Verification items for the finished model (mm, model axes). Face numbers are marked on the shaded views. A direction names the side the tool comes from. Give positions to 0.01 mm unless a question says otherwise; leave off trailing zeros.
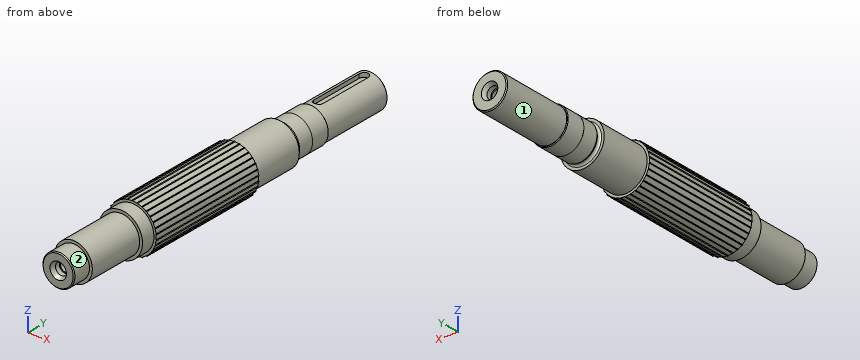
from build123d import *

# Parameters (mm, degrees)
F3_DEPTH        = 235.8934182005
F3_COPIES_COUNT = 30
F6_DEPTH        = 5
F7_SIZE         = 1.016
F10_D           = 10.5
F10_DEPTH       = 31.9574
F10_TIP         = 3.1545182499
F11_SIZE        = 0.762
F14_D           = 10.5
F14_DEPTH       = 31.9532
F14_TIP         = 3.1545182499


# Not quite as in the source:
# - a pattern or mirror of a feature is missing from the dataset's text; its kind, count and spacing are read off the source's solid


with BuildPart() as f1:
    # F0 (on Right) → F1 (revolve)
    with BuildSketch(Plane.YZ):
        with BuildLine():
            Line((59.3317817995, 23.876), (2.032, 23.876))
            Line((2.032, 23.876), (2.032, 27.1526))
            Line((2.032, 27.1526), (0, 27.1526))
            Line((0, 27.1526), (-135, 27.1526))
            Line((-135, 27.1526), (-135, 23.876))
            Line((-135, 23.876), (-150.24, 23.876))
            Line((-150.24, 23.876), (-150.24, 20.6375))
            Line((-150.24, 20.6375), (-213.3880182005, 20.6375))
            Line((-213.3880182005, 20.6375), (-213.3880182005, 17.5006))
            Line((-213.3880182005, 17.5006), (-233.8604182005, 17.5006))
            Line((-233.8604182005, 17.5006), (-233.8604182005, 9.0551))
            Line((-233.8604182005, 9.0551), (-229.4662182005, 6.5024))
            Line((-229.4662182005, 6.5024), (-224.3608182005, 6.5024))
            Line((-224.3608182005, 6.5024), (-224.3608182005, 0))
            Line((-224.3608182005, 0), (174.0127817995, 0))
            Line((174.0127817995, 0), (174.0127817995, 6.5024))
            Line((174.0127817995, 6.5024), (179.1181817995, 6.5024))
            Line((179.1181817995, 6.5024), (183.5123817995, 9.0551))
            Line((183.5123817995, 9.0551), (183.5123817995, 18.9992))
            Line((183.5123817995, 18.9992), (103.5023817995, 18.9992))
            Line((103.5023817995, 18.9992), (103.5023817995, 19.97075))
            Line((103.5023817995, 19.97075), (81.7853817995, 19.97075))
            Line((81.7853817995, 19.97075), (81.7853817995, 20.00758))
            Line((81.7853817995, 20.00758), (64.3216122695, 20.00758))
            Line((64.3216122695, 20.00758), (62.6845817995, 19.0624400175))
            ThreePointArc((62.6845817995, 19.0624400175), (60.4493817995, 19.0624400175), (59.3317817995, 20.99818))
            Line((59.3317817995, 20.99818), (59.3317817995, 23.876))
        make_face()
    revolve(axis=Axis((0, -25.1740182005, 0), (0, 1, 0)))

    # F2 (on face) → F3 (cut, through all)
    with BuildSketch(Plane(origin=(0, 2.032, 0), x_dir=(-1, 0, 0), z_dir=(0, 1, 0))):
        with BuildLine():
            Line((-0.442078818, 26.3868970263), (0, 27.1526))
            ThreePointArc((0, 27.1526), (-2.8382195517, 27.0038552162), (-5.6453429761, 26.5592505437))
            Line((-5.6453429761, 26.5592505437), (-5.0537260411, 25.9021933716))
            ThreePointArc((-5.0537260411, 25.9021933716), (-2.7585688627, 26.2460295319), (-0.442078818, 26.3868970263))
        make_face()
    f3 = extrude(amount=-F3_DEPTH, mode=Mode.SUBTRACT)

    # F3_copies: F3 ×30 about axis
    f3_copies_axis = Axis((0, 0, 0), (0, 1, 0))
    for i in range(1, F3_COPIES_COUNT):
        add(f3.rotate(f3_copies_axis, i * 360 / F3_COPIES_COUNT), mode=Mode.SUBTRACT)

    # F5 (on offset) → F6 (cut)
    with BuildSketch(Plane.XY.offset(18.9992)):
        with BuildLine():
            Line((-4.99999, 174.5207817995), (-4.99999, 113.5607817995))
            ThreePointArc((-4.99999, 113.5607817995), (0, 108.5607917995), (4.99999, 113.5607817995))
            Line((4.99999, 113.5607817995), (4.99999, 174.5207817995))
            ThreePointArc((4.99999, 174.5207817995), (0, 179.5207717995), (-4.99999, 174.5207817995))
        make_face()
    extrude(amount=-F6_DEPTH, mode=Mode.SUBTRACT)

    # F7
    f7_edges = [f1.edges().sort_by_distance(p)[0] for p in [
        (0, 183.512382, -18.9992),
        (0, -233.860418, -17.5006),
    ]]
    chamfer(f7_edges, length=F7_SIZE)

    # F10
    with Locations(Plane(origin=(0, 174.0127817995, 0), x_dir=(-1, 0, 0), z_dir=(0, 1, 0))):
        with Locations((0, 0)):
            Hole(F10_D / 2, depth=F10_DEPTH)
            with Locations((0, 0, -(F10_DEPTH + F10_TIP / 2))):  # 118° drill point
                Cone(0, F10_D / 2, F10_TIP, mode=Mode.SUBTRACT)

    # F11
    f11_edges = [f1.edges().sort_by_distance(p)[0] for p in [
        (0, 103.502382, -19.97075),
    ]]
    chamfer(f11_edges, length=F11_SIZE)

    # F14
    with Locations(Plane.XZ.offset(224.3608182005)):
        with Locations((0, 0)):
            Hole(F14_D / 2, depth=F14_DEPTH)
            with Locations((0, 0, -(F14_DEPTH + F14_TIP / 2))):  # 118° drill point
                Cone(0, F14_D / 2, F14_TIP, mode=Mode.SUBTRACT)


solid = f1.part
Item 1: Depth check by flat-ended pin: pin 1 (3.5 mm diameter, centred on y = 147, z = 16.5, fed in from -X); pin 2 (9.5 mm diameter, centred on x = 0, z = 0, fed in from -Y); pin 3 (1 mm diameter, centred on y = 22.5, z = -10.5, fed in from -X). Enter the tip coordinate at first touch or a pass-through.
Answer key:
pin 1: stops at x = -11.98
pin 2: stops at y = -192.11
pin 3: stops at x = -21.68
Item 2: Set-up check for the marked faces 1 and 2: record each of +Z, -Z, +X, -X, +Y, -Y from which the full face is reachable in a straight line by a thin tool's end or side.
Answer key:
face 1: +Y
face 2: -Y
Item 3: Scan lines: line 1 along X through (y, z) = (176.05, 0); line 2 along Z through (x, y) = (-16.5, 36.5); line 3 along X through (y, z) = (-70, 24.5). Record each from-to range of solid material in increasing order.
Answer key:
line 1: x = -19 to -6.5, 6.5 to 19
line 2: z = -17.26 to 17.26
line 3: x = -11.08 to -10.62, -9.81 to 9.81, 10.62 to 11.08
